from build123d import *

# Parameters (mm, degrees)
F0_R     = 1.1
F0_R_2   = 2
F1_DEPTH = 1.65
F2_R     = 2
F3_DEPTH = 3.85
F4_R     = 2
F4_R_2   = 1.9
F4_R_3   = 0.675
F5_DEPTH = 0.5
F6_DEPTH = 7


with BuildPart() as f1:
    # F0 (on Top) → F1 (new body)
    with BuildSketch(Plane.XY):
        with BuildLine():
            ThreePointArc((-13.040082, 13.43275), (-11.040082, 14.295292), (-9.040082, 13.43275))
            Line((-9.040082, 13.43275), (-9.040082, 18.645292))
            ThreePointArc((-9.040082, 18.645292), (-11.040082, 20.645292), (-13.040082, 18.645292))
            Line((-13.040082, 18.645292), (-13.040082, 13.43275))
        make_face()
        with Locations((-11.040082, 18.645292)):
            Circle(F0_R, mode=Mode.SUBTRACT)
        with BuildLine():
            Line((-16.188862, 6.263241), (-11.674669, 8.869512))
            ThreePointArc((-11.674669, 8.869512), (-13.421652, 10.170292), (-13.674669, 12.333613))
            Line((-13.674669, 12.333613), (-18.188862, 9.727343))
            ThreePointArc((-18.188862, 9.727343), (-18.920913, 6.995292), (-16.188862, 6.263241))
        make_face()
        with Locations((-17.188862, 7.995292)):
            Circle(F0_R, mode=Mode.SUBTRACT)
        with BuildLine():
            ThreePointArc((-10.405495, 8.869512), (-8.882813, 9.839803), (-8.290082, 11.545292))
            ThreePointArc((-8.290082, 11.545292), (-8.319088, 11.943654), (-8.405495, 12.333613))
            ThreePointArc((-8.405495, 12.333613), (-8.658512, 12.920292), (-9.040082, 13.43275))
            ThreePointArc((-9.040082, 13.43275), (-11.040082, 14.295292), (-13.040082, 13.43275))
            ThreePointArc((-13.040082, 13.43275), (-13.421652, 12.920292), (-13.674669, 12.333613))
            ThreePointArc((-13.674669, 12.333613), (-13.421652, 10.170292), (-11.674669, 8.869512))
            ThreePointArc((-11.674669, 8.869512), (-11.040082, 8.795292), (-10.405495, 8.869512))
        make_face()
        with Locations((-11.040082, 11.545292)):
            Circle(F0_R_2, mode=Mode.SUBTRACT)
        with BuildLine():
            ThreePointArc((-8.405495, 12.333613), (-8.319088, 11.943654), (-8.290082, 11.545292))
            ThreePointArc((-8.290082, 11.545292), (-8.882813, 9.839803), (-10.405495, 8.869512))
            Line((-10.405495, 8.869512), (-5.891302, 6.263241))
            ThreePointArc((-5.891302, 6.263241), (-3.159251, 6.995292), (-3.891302, 9.727343))
            Line((-3.891302, 9.727343), (-8.405495, 12.333613))
        make_face()
        with Locations((-4.891302, 7.995292)):
            Circle(F0_R, mode=Mode.SUBTRACT)
    extrude(amount=F1_DEPTH)

    # F2 (on face) → F3 (join)
    with BuildSketch(Plane.XY.offset(1.65)):
        with BuildLine():
            ThreePointArc((-10.405495, 8.869512), (-8.882813, 9.839803), (-8.290082, 11.545292))
            ThreePointArc((-8.290082, 11.545292), (-8.319088, 11.943654), (-8.405495, 12.333613))
            ThreePointArc((-8.405495, 12.333613), (-8.658512, 12.920292), (-9.040082, 13.43275))
            ThreePointArc((-9.040082, 13.43275), (-11.040082, 14.295292), (-13.040082, 13.43275))
            ThreePointArc((-13.040082, 13.43275), (-13.421652, 12.920292), (-13.674669, 12.333613))
            ThreePointArc((-13.674669, 12.333613), (-13.421652, 10.170292), (-11.674669, 8.869512))
            ThreePointArc((-11.674669, 8.869512), (-11.040082, 8.795292), (-10.405495, 8.869512))
        make_face()
        with Locations((-11.040082, 11.545292)):
            Circle(F2_R, mode=Mode.SUBTRACT)
    extrude(amount=F3_DEPTH)

    # F4 (on face) → F5 (join)
    with BuildSketch(Plane.XY.offset(5.5)):
        with Locations((-11.040082, 11.545292)):
            Circle(F4_R)
        with Locations((-11.040082, 11.545292)):
            Circle(F4_R_2, mode=Mode.SUBTRACT)
        with Locations((-11.040082, 11.545292)):
            Circle(F4_R_2)
        with Locations((-11.040082, 11.545292)):
            Circle(F4_R_3, mode=Mode.SUBTRACT)
    extrude(amount=-F5_DEPTH)

    # F4 (on face) → F6 (join)
    with BuildSketch(Plane.XY.offset(5.5)):
        with Locations((-11.040082, 11.545292)):
            Circle(F4_R_2)
        with Locations((-11.040082, 11.545292)):
            Circle(F4_R_3, mode=Mode.SUBTRACT)
    extrude(amount=F6_DEPTH)


solid = f1.part
The listing builds one solid part. Answer for the finished solid, in the listing's coordinates (mm). A direction names the side the tool comes from. Give positions to 0.01 mm unless a question says otherwise; leave off trailing zeros. Loops run counter-clockwise (first coordinate to the right, second up) from the corner with the lowest first, then second, coordinate; pieces in that order, holes last. Notation, with made-up numbers: (5, 38.25) - (43, 38.25) arc R10 cw to (43, 42.25) - close; hole circle Ø8 at (19.5, 45.25). An arc over 180 degrees is marked (long way). Use one line per item in the form item = value.
1. Section D-D on y = 7.5 is taken. Give the vertices of the cut face in (x, z), then the cut area to 3 significant figures.
Calculated:
outline = (-19.13, 0) - (-18.17, 0) - (-18.17, 1.65) - (-19.13, 1.65) - close; (-16.21, 0) - (-14.05, 0) - (-14.05, 1.65) - (-16.21, 1.65) - close; (-8.03, 0) - (-5.87, 0) - (-5.87, 1.65) - (-8.03, 1.65) - close; (-3.91, 0) - (-2.95, 0) - (-2.95, 1.65) - (-3.91, 1.65) - close
area = 10.3 mm^2
2. Find the intervals of material crossed by line 1 along Z through (x, y) = (-12, 12.75); line 2 along Z through (x, y) = (-16.75, 10.5); line 3 along X through (y, z) = (15.25, 0.5), in increasing order. Write a range as [from, to].
Calculated:
line_1 = [5, 12.5]
line_2 = [0, 1.65]
line_3 = [-13.04, -9.04]
3. Section B-B on x = -17.5 is taken. Give the vertices of the cut face in (y, z).
Calculated:
outline = (6.02, 0) - (6.94, 0) - (6.94, 1.65) - (6.02, 1.65) - close; (9.05, 0) - (10.13, 0) - (10.13, 1.65) - (9.05, 1.65) - close
4. Section A-A on z = 4 is taken. Give the vertices of the cut face in (x, y), then the cut area to 3 significant figures.
Calculated:
outline = (-13.67, 12.33) arc R2.75 ccw to (-11.67, 8.87) arc R2.75 ccw to (-10.41, 8.87) arc R2.75 ccw to (-8.29, 11.55) arc R2.75 ccw to (-8.41, 12.33) arc R2.75 ccw to (-9.04, 13.43) arc R2.75 ccw to (-13.04, 13.43) arc R2.75 ccw to start; hole circle Ø4 at (-11.04, 11.55)
area = 11.2 mm^2
5. The mould has two halves that part along Y. Classify faces 1 (the face through (-10.417, 11.287, 8.698)), 2 (the face through (-10.02, 13.15, 8.95)), 3 (the face through (-9, 12, 5.5)): pulls with the +Y half, pulls with the -Y half, needs draft (parallel to the pull), parting line crosses it, or undercut.
Calculated:
face_1 = undercut
face_2 = parting line crosses it
face_3 = needs draft
6. Section C-C on y = 11.75 is taken. Give the vertices of the cut face in (x, z).
Calculated:
outline = (-14.69, 0) - (-13.03, 0) - (-13.03, 5) - (-11.68, 5) - (-11.68, 12.5) - (-12.93, 12.5) - (-12.93, 5.5) - (-13.78, 5.5) - (-13.78, 1.65) - (-14.69, 1.65) - close; (-10.4, 5) - (-9.05, 5) - (-9.05, 0) - (-7.39, 0) - (-7.39, 1.65) - (-8.3, 1.65) - (-8.3, 5.5) - (-9.15, 5.5) - (-9.15, 12.5) - (-10.4, 12.5) - close
7. Given pin 1 Ø3 at (x, y) = (-11.04, 18.65) entering from -Z; pin 2 Ø5 at (x, y) = (-6.5, 9) entering from +Z; pin 3 Ø2 at (x, y) = (-17.19, 8) entering from +Z; pin 4 Ø5 at (x, z) = (-7, 9) entering from +Y, each flat-ended and moving along its own axis, determine where each tip first touches the part or whether it passes through.
Calculated:
pin_1 = 0
pin_2 = 5.5
pin_3 = through
pin_4 = 12.66
8. Which of the six approach directions +Z, -Z, +X, -X, +Y, -Y give full straight-line access (tool end or side, diameter ignored) to faces 4 (the face through (-13.04, 16, 1)), 5 (the face through (-13.96, 7.55, 0.81)), 6 (the face through (-10, 12, 5))?
Calculated:
face_4 = +Z, -Z, -X, +Y
face_5 = +Z, -Z, -Y
face_6 = -Z
